CAD build for the part. Positions are in the model's coordinates, mm. A direction names the side the tool comes from. Give positions to 0.01 mm unless a question says otherwise; leave off trailing zeros. Order: outer loops, then holes, each group sorted by start corner. A loop starts at its lowest first (then second) coordinate and runs counter-clockwise, first axis right, second up. Notation, with made-up numbers: (64, -9) -> (92, -9) arc R24 cw to (92, 23) -> close; hole circle Ø3 at (29, 8). An arc over 180 degrees is marked (long way). Use one line per item in the form item = value. Start each with the question number.
1) Cut at D-D, the plane y = -19.5. Give the cut face in (x, z).
2) Probe line 1 (Y direction, x = -30.95, z = -7.5); line 2 (X direction, y = 2.5, z = -7.5); line 3 (X direction, y = -10, z = -7.75). List the from-to ranges inside material, lowest first.
3) Mould opens along Y. For faces 1 (the face through (-13, -9, -15)), 2 (the face through (-24, -9, -7)), 3 (the face through (-15, -21, -8)) say: pulls with the +Y half, pulls with the -Y half, needs draft (parallel to the pull), parting line crosses it, or undercut.
4) Cut at A-A, the plane x = -15.5. Give the cut face in (y, z), and give its area (3 significant figures).
5) Cut at B-B, the plane x = -22. Give the cut face in (y, z) (3 decimals), and give its area (3 significant figures).
6) Tool access for faces 4 (the face through (-23, -29, -4.325)), 5 (the face through (-15, 7.4, -5.7)), 6 (the face through (-13, 9, -9)), 7 (the face through (-9.697, 12.031, -9.896)): list every direction of +Z, -Z, +X, -X, +Y, -Y with a clear straight run to the whole face (end or side of a thin tool).
7) Drop flat-ended pins along their axis: P1, Ø4, axis at y = -30.25, z = -7.5, coming from the -X side; P2, Ø1, axis at y = 9.5, z = -8, coming from the -X side; P3, Ø5, axis at x = -7.5, z = -8, coming from the +Y side; P4, Ø1, axis at x = -24.5, z = -5.5, coming from the -Y side. Give the stop position or say it passes through.
8) Cut at C-C, the plane z = -12.5. Give the cut face in (x, y).
Autodesk Inventor part; units mm, degrees
ref_plane "YZ Plane" through (0, 0, 0) normal (1, 0, 0) x (0, 1, 0)
ref_plane "XZ Plane" through (0, 0, 0) normal (0, 1, 0) x (-1, 0, 0)
ref_plane "XY Plane" through (0, 0, 0) normal (0, 0, 1) x (1, 0, 0)
sketch "Base Profile" plane through (0, 0, 0) normal (0, 1, 0) x (-1, 0, 0)
  line L0 (0, 0) -> (15, 0)
  line L1 (15, 0) -> (15, -15)
  line L2 (15, -15) -> (0, -15)
  line L3 (0, -15) -> (0, 0)
  line L4 (15, 0) -> (32, 0)
  line L5 (32, 0) -> (32, -15)
  line L6 (32, -15) -> (15, -15)
  line L7 (15, -15) -> (15, 0)
  dimension "d164" = 15
  dimension "d165" = 15
  dimension "d166" = 17
  dimension "d167" = 15
extrude "Stock" add sketch "Base Profile" against normal blind 33
extrude "Extrusion Post" add sketch "Base Profile" along normal blind 15 contours L0 L1 L2 L3
sketch "Sketch27" plane through (0, -33, -15) normal (0, 0, -1) x (-1, 0, 0)
  line L0 (0, 0) -> (0, 48)
  line L1 (32, 0) -> (0, 0)
  line L2 (32, 33) -> (32, 0)
  line L3 (15, 33) -> (32, 33)
  line L4 (15, 33) -> (15, 48)
  line L5 (0, 48) -> (15, 48)
  line L6 (0, 16.5) -> (32, 16.5)
  line L7 (0, 7.5) -> (32, 7.5)
  line L8 (15, 33) -> (15, 0)
  point P0 (15, 16.5)
  point P1 (15, 7.5)
  dimension "d247" = 16.5
  dimension "d290" = 7.5
extrude "Lower Half Cut" cut sketch "Sketch27" against normal through all contours L8 L6 L2 L7
sketch "Bottom Profile" plane through (-35, -33, -15) normal (0, -1, 0) x (1, 0, 0)
  line L0 (13.5, 7.5) -> (9.5, 7.5) construction
  line L1 (13.5, 10.675) -> (9.5, 10.675)
  line L2 (9.5, 4.325) -> (13.5, 4.325)
  arc A0 (13.5, 4.325) -> (13.5, 10.675) centre (13.5, 7.5) ccw
  arc A1 (9.5, 10.675) -> (9.5, 4.325) centre (9.5, 7.5) ccw
  line L3 (3, 15) -> (3, 0)
  line L4 (35, 15) -> (3, 15)
  point P0 (11.5, 7.5)
  dimension "d291" = 4
  dimension "d292" = 6.35
  dimension "d293" = 6.5
  dimension "d294" = 7.5
extrude "Slot Cut" cut sketch "Bottom Profile" against normal blind 24
sketch "Front Hole Pattern" plane through (0, -33, 0) normal (1, 0, 0) x (0, 0, -1)
  line L0 (0, 0) -> (0, 48)
  circle A0 centre (7.5, 40.5) radius 3.175
  line L1 (0, 48) -> (15, 48)
  dimension "d317" = 6.35
  dimension "d318" = 7.5
  dimension "d319" = 7.5
sketch "Rear Hole Patttern" plane through (-32, -33, -15) normal (-1, 0, 0) x (0, 0, 1)
  line L0 (15, 7.5) -> (0, 7.5)
  line L1 (0, 7.5) -> (0, 0)
  line L2 (15, 0) -> (0, 0)
  line L3 (15, 7.5) -> (15, 0)
  line L4 (0, 5.5) -> (15, 5.5) construction
  circle A0 centre (7.5, 2.75) radius 1.5
  line L5 (0, 16.5) -> (15, 16.5)
  line L6 (15, 33) -> (15, 16.5)
  line L7 (0, 33) -> (15, 33)
  line L8 (0, 33) -> (0, 16.5)
  line L9 (0, 18.5) -> (15, 18.5) construction
  line L10 (0, 24) -> (15, 24) construction
  circle A1 centre (7.5, 21.25) radius 1.5
  dimension "d328" = 2
  dimension "d329" = 7.5
  dimension "d330" = 3
  dimension "d331" = 7.5
  dimension "d332" = 2.75
  dimension "d350" = 2
  dimension "d351" = 7.5
  dimension "d352" = 3
  dimension "d353" = 2.75
hole "Rear Holes" at (-32, -30.25, -7.5) at (-32, -11.75, -7.5) direction (1, 0, 0) diameter 2.459 depth 13.6652 tip angle 118
hole "Front Mounting Hole" at (0, 7.5, -7.5) direction (-1, 0, 0) diameter 3.2004 end through all counterbore diameter 6.5024 counterbore depth 13
sketch "Sketch33" plane through (0, 15, 0) normal (0, 1, 0) x (1, 0, 0)
  line L0 (-15, 15) -> (-15, 0)
  line L1 (-15, 0) -> (0, 0)
  line L2 (0, 0) -> (0, 15)
  line L3 (0, 15) -> (-15, 15)
  circle A0 centre (-7.5, 7.5) radius 3.175
  dimension "d340" = 6.35
  dimension "d341" = 7.5
  dimension "d342" = 7.5
hole "Top Mounting Hole" at (-7.5, 15, -7.5) direction (0, -1, 0) diameter 3.2004 end through all counterbore diameter 6.5024 counterbore depth 18
fillet "Fillet2" radius 6.35 2 edges at (-32, -29.25, 0) (-32, -8.25, 0)
equation "\"d164\" = extrusionWidth"
equation "\"d165\" = extrusionWidth"
equation "\"d166\" = idlerLength"
equation "\"d167\" = d165"
equation "\"d168\" = extrusionOffset"
equation "\"extrusionWidth\" = 15"
equation "\"idlerLength\" = 17"
equation "\"bearingOffsetFromBottom\" = 7.5"
equation "\"extrusionOffset\" = 33"
equation "\"bearingStackHeight\" = 9"
equation "\"bearingSlotLength\" = 4"
equation "\"bearingClearance\" = 13"
equation "\"pinSupportLength\" = 2"
properties part number "A Idler" material "Aluminum 6061"
Result:
q1.outline = (-15, -15) -> (0, -15) -> (0, 0) -> (-15, 0) -> close; hole circle Ø3.2 at (-7.5, -7.5)
q2.line_1 = -33 to -31.48, -29.02 to -25.5, -16.5 to -12.98, -10.52 to 0
q2.line_2 = -15 to -10.75, -4.25 to 0
q2.line_3 = -32 to -28.67, -18.33 to -9.08, -5.92 to 0
q3.face_1 = needs draft
q3.face_2 = pulls with the -Y half
q3.face_3 = undercut
q4.outline = (-33, -15) -> (-25.5, -15) -> (-25.5, 0) -> (-33, 0) -> close; (-16.5, -15) -> (0, -15) -> (0, 0) -> (-16.5, 0) -> close
q4.area = 360 mm²
q5.outline = (-33, -15) -> (-25.5, -15) -> (-25.5, -10.675) -> (-33, -10.675) -> close; (-33, -4.325) -> (-25.5, -4.325) -> (-25.5, 0) -> (-33, 0) -> close; (-16.5, -15) -> (0, -15) -> (0, 0) -> (-16.5, 0) -> (-16.5, -4.325) -> (-9, -4.325) -> (-9, -10.675) -> (-16.5, -10.675) -> close
q5.area = 265 mm²
q6.face_4 = -Y
q6.face_5 = +Z, -Z, -X, +Y
q6.face_6 = +X
q6.face_7 = +Y
q7.P1 = -32
q7.P2 = -15
q7.P3 = -3
q7.P4 = -9
q8.outline = (-32, -33) -> (0, -33) -> (0, 15) -> (-15, 15) -> (-15, 0) -> (-32, 0) -> (-32, -16.5) -> (-15, -16.5) -> (-15, -25.5) -> (-32, -25.5) -> close
